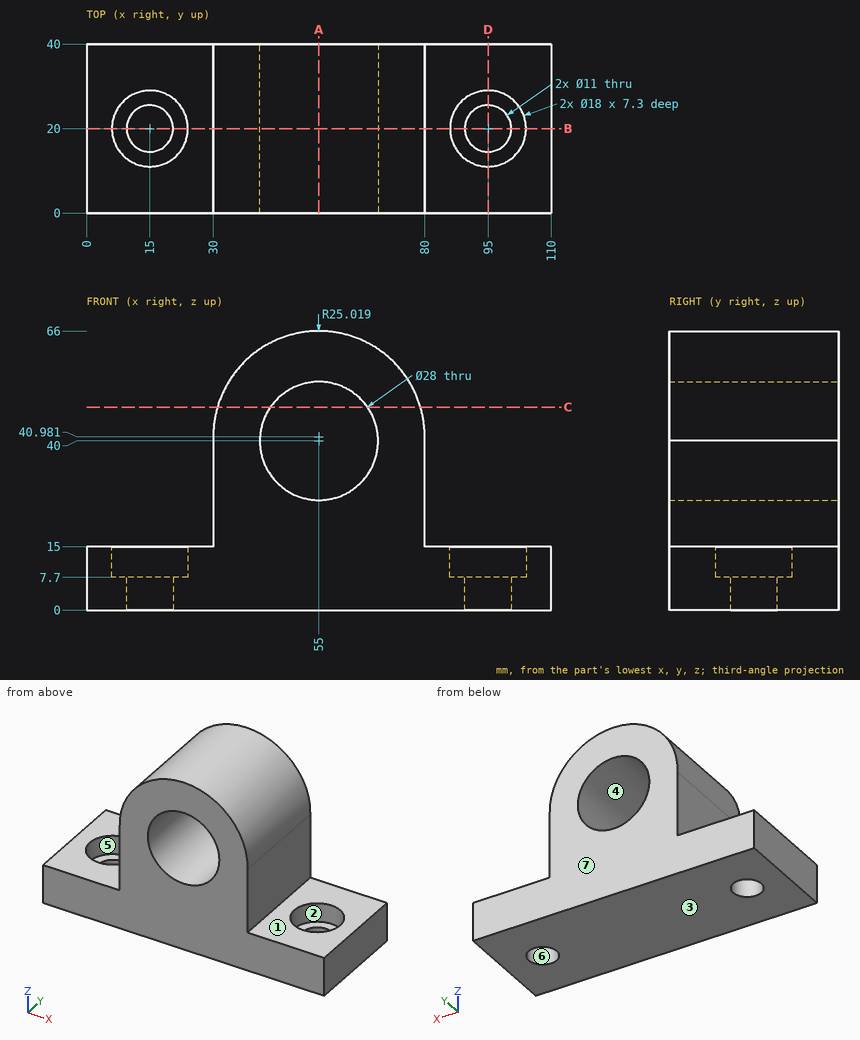
Answer from the drawing. Dimensions are ordinates in mm from the lowest x, y and z of the part. A direction names the side the tool comes from. Round coordinates to 2 decimals unless told otherwise and drop trailing zeros. Write each loop counter-clockwise with the first axis right and the second up, starting at its lowest first coordinate (ties: lowest second). Pieces come first, ordered by that corner, then holes. Notation, with made-up numbers: M 15,-35.5 L 32,-35.5 A12 ccw 32,-18.5 Z; hole C 27.25,-34.5 d4. An arc over 180 degrees is marked long. Write each question's results on one line, items separated by ' | '. Start each with the question number.
Item 1: Find section C-C on z = 48. Write down the section's boundary in (x, y).
Item 2: Find section D-D on x = 95. Write down the section's boundary in (y, z).
Item 3: Given pin 1 Ø8 at (x, y) = (17.5, 29) entering from +Z; pin 2 Ø9 at (x, y) = (15, 20) entering from -Z; pin 3 Ø3 at (y, z) = (35.5, 26.5) entering from +X; pin 4 Ø1.5 at (y, z) = (31.5, 37.5) entering from -X, each flat-ended and moving along its own axis, determine where each tip first touches the part or whether it passes through.
Item 4: Straight lines are drawn through the part: probe 1 along Y at (x, z) = (95, 4.5); probe 2 along X at (y, z) = (13, 10); probe 3 along Y at (x, z) = (95, 11). For each, find the intervals that lie inside material, in ascending order.
Item 5: The mould has two halves that part along Y. Classify the marked faces 4, 5, 6 and 7: +Y half, -Y half, draft (parallel to the pull), parting line (faces both ways), or undercut.
Item 6: Find section B-B on y = 20. Write down the section's boundary in (x, z), and give its area (3 significant figures).
Item 7: Find section A-A on x = 55. Write down the section's boundary in (y, z).
Item 8: Which of the six approach directions +Z, -Z, +X, -X, +Y, -Y give full straight-line access (tool end or side, diameter ignored) to the marked faces 1, 2 and 3?
Answer block:
1) outline: M 30.99,0 L 43.51,0 L 43.51,40 L 30.99,40 Z; M 66.49,0 L 79.01,0 L 79.01,40 L 66.49,40 Z
2) outline: M 0,0 L 14.5,0 L 14.5,7.7 L 11,7.7 L 11,15 L 0,15 Z; M 25.5,0 L 40,0 L 40,15 L 29,15 L 29,7.7 L 25.5,7.7 Z
3) pin 1: stops at z = 15 | pin 2: passes through | pin 3: stops at x = 80 | pin 4: stops at x = 30
4) probe 1: y = 0 to 14.5, 25.5 to 40 | probe 2: x = 0 to 9.34, 20.66 to 89.34, 100.66 to 110 | probe 3: y = 0 to 11, 29 to 40
5) face 4: draft | face 5: undercut | face 6: undercut | face 7: +Y half
6) outline: M 0,0 L 9.5,0 L 9.5,7.7 L 6,7.7 L 6,15 L 0,15 Z; M 20.5,0 L 89.5,0 L 89.5,7.7 L 86,7.7 L 86,15 L 80,15 L 80,40 A25.02 ccw long 30,40 L 30,15 L 24,15 L 24,7.7 L 20.5,7.7 Z; M 100.5,0 L 110,0 L 110,15 L 104,15 L 104,7.7 L 100.5,7.7 Z; hole C 55,40 d28 | area: 2,880 mm²
7) outline: M 0,0 L 40,0 L 40,26 L 0,26 Z; M 0,54 L 40,54 L 40,66 L 0,66 Z
8) face 1: +Z, +X, +Y, -Y | face 2: +Z | face 3: -Z, +X, -X, +Y, -Y
